```python
from build123d import *

# Parameters (mm, degrees)
F0_W     = 101.6
F0_H     = 12.7
F1_DEPTH = 101.6
F3_D     = 14.2875
F4_W     = 239.776
F4_H     = 152.4
F5_DEPTH = 6.35
F6_SIZE  = 25.4
F7_SIZE  = 127


with BuildPart() as f1:
    # F0 (on Front) → F1 (new body, symmetric)
    with BuildSketch(Plane.XZ):
        with Locations((50.8, 6.35)):
            Rectangle(F0_W, F0_H)
    extrude(amount=F1_DEPTH, both=True)

    # F3 (through all)
    with Locations(Plane.XY.offset(12.7)):
        with Locations((25.4, -76.2), (76.2, -76.2), (76.2, 76.2), (25.4, 76.2)):
            Hole(F3_D / 2)

    # F4 (on Front) → F5 (join, symmetric)
    with BuildSketch(Plane.XZ):
        with Locations((-18.288, -76.2)):
            Rectangle(F4_W, F4_H)
    extrude(amount=F5_DEPTH, both=True)

    # F6
    f6_edges = [f1.edges().sort_by_distance(p)[0] for p in [
        (-138.176, 0, 0),
    ]]
    chamfer(f6_edges, length=F6_SIZE)

    # F7
    f7_edges = [f1.edges().sort_by_distance(p)[0] for p in [
        (101.6, 0, -152.4),
    ]]
    chamfer(f7_edges, length=F7_SIZE)


solid = f1.part
```
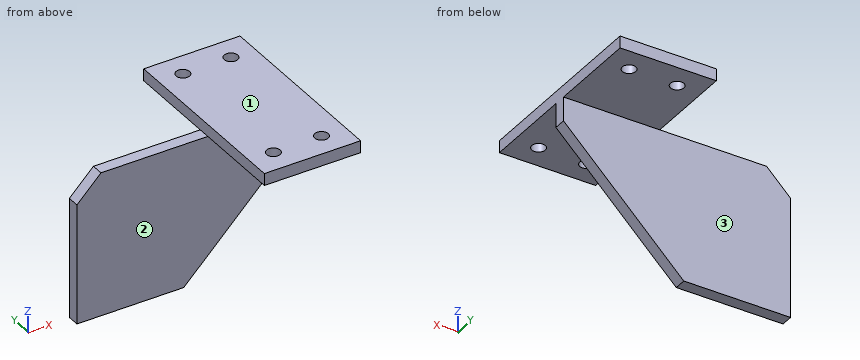
CAD build for the part. Positions are in the model's coordinates, mm. Face numbers are marked on the shaded views. A direction names the side the tool comes from. Round coordinates to 2 decimals unless told otherwise and drop trailing zeros. Order: outer loops, then holes, each group sorted by start corner. A loop starts at its lowest first (then second) coordinate and runs counter-clockwise, first axis right, second up.
Q1. Slice it at A-A (x = 76.2). Write the cut outline in (y, z), and give its area (3 significant figures).
Q2. Which spindle directions (+Z, -Z, +X, -X, +Y, -Y) get a long thin tool onto all of the face, cutting with end or side? Do the marked faces 1, 2 and 3. Say none if no direction does.
Q3. Slice it at C-C (x = 25.4). Write the cut outline in (y, z), and give its area (3 significant figures).
Q4. Wall check: L1, parallel to Y at x = 25, z = 7; L2, parallel to X at y = 76, z = 9; L3, parallel to Y at x = -127, z = -80.5. Give the ranges that are in metal, low to high.
Q5. Slice it at B-B (y = 76.2). Write the cut outline in (x, z).
Q6. Drop flat-ended pins along their axis: pin 1 (6.5 mm diameter, centred on x = -75.5, y = -2, fed in from +Z); pin 2 (12 mm diameter, centred on x = -54.5, z = -88, fed in from +Y); pin 3 (23 mm diameter, centred on x = 25.4, y = 76.2, fed in from -Z); pin 4 (13 mm diameter, centred on x = 76.2, y = -76.2, fed in from +Z). Give the stop position or say it passes through.
Q7. Slice it at D-D (y = -26.5). Write the cut outline in (x, z).
Results below:
1. outline: (-101.6, 0) - (-83.34, 0) - (-83.34, 12.7) - (-101.6, 12.7) - close; (-69.06, 0) - (-6.35, 0) - (-6.35, -50.8) - (6.35, -50.8) - (6.35, 0) - (69.06, 0) - (69.06, 12.7) - (-69.06, 12.7) - close; (83.34, 0) - (101.6, 0) - (101.6, 12.7) - (83.34, 12.7) - close
1. area: 2,860 mm2
2. face 1: +Z, +X, -X, +Y, -Y
2. face 2: -Z, +X, -X, -Y
2. face 3: -Z, +X, -X, +Y
3. outline: (-101.6, 0) - (-83.34, 0) - (-83.34, 12.7) - (-101.6, 12.7) - close; (-69.06, 0) - (-6.35, 0) - (-6.35, -101.6) - (6.35, -101.6) - (6.35, 0) - (69.06, 0) - (69.06, 12.7) - (-69.06, 12.7) - close; (83.34, 0) - (101.6, 0) - (101.6, 12.7) - (83.34, 12.7) - close
3. area: 3,510 mm2
4. L1: y = -101.6 to -83.33, -69.07 to 69.07, 83.33 to 101.6
4. L2: x = 0 to 18.26, 32.54 to 69.06, 83.34 to 101.6
4. L3: y = -6.35 to 6.35
5. outline: (0, 0) - (18.26, 0) - (18.26, 12.7) - (0, 12.7) - close; (32.54, 0) - (69.06, 0) - (69.06, 12.7) - (32.54, 12.7) - close; (83.34, 0) - (101.6, 0) - (101.6, 12.7) - (83.34, 12.7) - close
6. pin 1: stops at z = 0
6. pin 2: stops at y = 6.35
6. pin 3: stops at z = 0
6. pin 4: passes through
7. outline: (0, 0) - (101.6, 0) - (101.6, 12.7) - (0, 12.7) - close
